CAD build for the part. Positions are in the model's coordinates, mm. A direction names the side the tool comes from. Give positions to 0.01 mm unless a question says otherwise; leave off trailing zeros. Loops run counter-clockwise (first coordinate to the right, second up) from the corner with the lowest first, then second, coordinate; pieces in that order, holes last.
Item 1: Probe probe 1 along Z at (x, y) = (19, 122.5); probe 2 along X at (y, z) = (93, -55); probe 3 along Y at (x, z) = (122, -82.5). List the from-to ranges inside material, lowest first.
Item 2: Saw through at B-B on y = 73.5. Give the cut face in (x, z), plus the area to 3 significant figures.
Item 3: Which spindle directions (+Z, -Z, +X, -X, +Y, -Y) get a long thin tool onto all of the face, cutting with end or side? Do faces 1 (the flat face through (88, 125, 0)), 2 (the flat face through (88, 131, -2.54)). Say none if no direction does.
Item 4: Saw through at D-D on y = 161. Give the cut face in (x, z).
Item 5: Drop a flat-ended pin along its axis: P1, Ø6, axis at x = 65.5, z = -87, coming from the +Y side. Give the stop position or say it passes through.
Item 6: Mould opens along Z. For faces 3 (the flat face through (88, 125, -127)), 4 (the flat face through (177.8, 125, -61)), 5 (the flat face through (88, 131, -124.46)) say: released by +Z, released by -Z, zero draft, split by the parting line, or undercut.
Item 7: Saw through at C-C on x = 149. Give the cut face in (y, z).
Item 8: Saw through at A-A on z = -39. Give the cut face in (x, y), plus the area to 3 significant figures.
from build123d import *

# Parameters (mm, degrees)
SKETCH1_W           = 177.8
SKETCH1_H           = 127
BOSS_EXTRUDE1_DEPTH = 254
SKETCH2_W           = 172.72
SKETCH2_H           = 121.92
CUT_EXTRUDE1_DEPTH  = 248.92
FILLET2_R           = 2.54
FILLET3_START       = 95.25
FILLET3_DEPTH       = 159.75


with BuildPart() as part:
    # Sketch1 → Boss-Extrude1 (new body)
    with BuildSketch(Plane(origin=(0, 0, 0), x_dir=(1, 0, 0), z_dir=(0, 1, 0))):
        with Locations((88.9, 63.5)):
            Rectangle(SKETCH1_W, SKETCH1_H)
    extrude(amount=BOSS_EXTRUDE1_DEPTH)

    # Sketch2 → Cut-Extrude1 (cut)
    with BuildSketch(Plane(origin=(0, 254, 0), x_dir=(1, 0, 0), z_dir=(0, 1, 0))):
        with Locations((88.9, 63.5)):
            Rectangle(SKETCH2_W, SKETCH2_H)
    extrude(amount=-CUT_EXTRUDE1_DEPTH, mode=Mode.SUBTRACT)

    # Fillet2
    fillet2_edges = [part.edges().sort_by_distance(p)[0] for p in [
        (0, 127, -127),
        (177.8, 127, -127),
    ]]
    fillet(fillet2_edges, radius=FILLET2_R)

    # Fillet3: read off the stored shape, not the designer's step
    # Fillet3 outline → Fillet3 (cut)
    with BuildSketch(Plane(origin=(0, 0, 0), x_dir=(1, 0, 0), z_dir=(0, 1, 0)).offset(FILLET3_START)):
        with BuildLine():
            Line((0, 0), (2.54, 0))
            ThreePointArc((2.54, 0), (0.743948776, 0.743948776), (0, 2.54))
            Line((0, 2.54), (0, 0))
        make_face()
        with BuildLine():
            ThreePointArc((177.8, 2.54), (177.056051224, 0.743948776), (175.26, 0))
            Line((175.26, 0), (177.8, 0))
            Line((177.8, 0), (177.8, 2.54))
        make_face()
    extrude(amount=FILLET3_DEPTH, mode=Mode.SUBTRACT)


solid = part.part
Results below:
1. probe 1: z = -127 to -124.46, -2.54 to 0
1. probe 2: x = 0 to 2.54, 175.26 to 177.8
1. probe 3: y = 0 to 5.08
2. outline: (0, -124.46) arc R2.54 ccw to (2.54, -127) - (175.26, -127) arc R2.54 ccw to (177.8, -124.46) - (177.8, 0) - (0, 0) - close; hole (2.54, -124.46) - (175.26, -124.46) - (175.26, -2.54) - (2.54, -2.54) - close
2. area: 1,520 mm2
3. face 1: +Z, +X, -X, +Y, -Y
3. face 2: +Y
4. outline: (0, -124.46) arc R2.54 ccw to (2.54, -127) - (175.26, -127) arc R2.54 ccw to (177.8, -124.46) - (177.8, -2.54) arc R2.54 ccw to (175.26, 0) - (2.54, 0) arc R2.54 ccw to (0, -2.54) - close; hole (2.54, -124.46) - (175.26, -124.46) - (175.26, -2.54) - (2.54, -2.54) - close
5. P1: stops at y = 5.08
6. face 3: released by -Z
6. face 4: zero draft
6. face 5: undercut
7. outline: (0, -127) - (254, -127) - (254, -124.46) - (5.08, -124.46) - (5.08, -2.54) - (254, -2.54) - (254, 0) - (0, 0) - close
8. outline: (0, 0) - (177.8, 0) - (177.8, 254) - (175.26, 254) - (175.26, 5.08) - (2.54, 5.08) - (2.54, 254) - (0, 254) - close
8. area: 2,170 mm2
